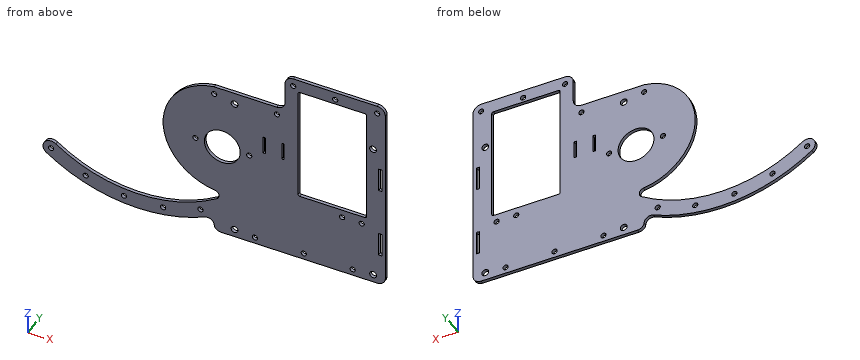
Autodesk Inventor part; units mm, degrees
ref_plane "YZ Plane" through (0, 0, 0) normal (1, 0, 0) x (0, 1, 0)
ref_plane "XZ Plane" through (0, 0, 0) normal (0, 1, 0) x (-1, 0, 0)
ref_plane "XY Plane" through (0, 0, 0) normal (0, 0, 1) x (1, 0, 0)
sketch "Sketch1" plane through (0, 0, 0) normal (0, 1, 0) x (-1, 0, 0)
  arc A0 (-0.3814, 2.9757) -> (-3, 0) centre (0, 0) ccw
  circle A1 centre (-5, 35) radius 11
  arc A2 (-0.3814, 2.9757) -> (0, 75) centre (-5, 39.0133) ccw
  line L0 (-105, 0) -> (0, 0) construction
  line L1 (-3, 0) -> (-105, 0) construction
  arc A3 (-3, 0) -> (-0.3814, -2.9757) centre (0, 0) ccw
  arc A4 (-1.6619, -2.4976) -> (97.0992, -0.9275) centre (46.5785, 70) ccw
  arc A5 (102.9008, -9.0725) -> (97.0992, -0.9275) centre (100, -5) ccw
  line L2 (0, 0) -> (100, 0) construction
  arc A6 (5.6849, -18.0476) -> (102.9008, -9.0725) centre (46.5785, 70) ccw
  line L3 (0, 75) -> (0, 0) construction
  line L4 (0, 0) -> (0, -15.1769) construction
  line L5 (0, 0) -> (-105, 0) construction
  line L6 (0, 75) -> (-105, 75)
  line L7 (-105, 75) -> (-105, -25)
  line L8 (0, -21.6754) -> (0, -21)
  line L9 (-4, -25) -> (-105, -25)
  arc A7 (5.6849, -18.0476) -> (0, -21.6754) centre (4, -21.6754) ccw
  arc A8 (-4, -25) -> (0, -21) centre (-4, -21) ccw
  point P0 (-5, -39.0133)
  point P1 (0, -25)
  dimension "d0" = 6
  dimension "d7" = 22
  dimension "d13" = 5
  dimension "d47" = 10
  dimension "d49" = 100
  dimension "d68" = 70
  dimension "d71" = 0
  dimension "d75" = 105
  dimension "d76" = 4
  dimension "d77" = 4
  dimension "d101" = 100
  dimension "d105" = 75
  dimension "d106" = 35
  dimension "d107" = 5
extrude "Extrusion1" add sketch "Sketch1" along normal blind 2
sketch "Szkic5" plane through (0, 2, 0) normal (0, 1, 0) x (1, 0, 0)
  circle A0 centre (12.5, 20) radius 2.1
  circle A1 centre (97.5, 20) radius 2.1
  circle A2 centre (12.5, -67.5) radius 2.1
  circle A3 centre (97.5, -67.5) radius 2.1
  line L0 (12.5, 20) -> (97.5, 20) construction
  line L1 (97.5, -67.5) -> (97.5, 20) construction
  line L2 (12.5, -67.5) -> (97.5, -67.5) construction
  line L3 (0, -75) -> (105, -75) construction
  line L4 (105, -75) -> (105, 25) construction
  line L5 (105, 25) -> (4, 25) construction
  line L6 (0, 21) -> (0, 21.6754) construction
  line L7 (12.5, 20) -> (12.5, -67.5) construction
  point P0 (0, 0)
  dimension "d84" = 7.5
  dimension "d85" = 7.5
  dimension "d88" = 4.2
  dimension "d89" = 85
  dimension "d109" = 87.5
extrude "Wyciągnięcie proste4" cut sketch "Szkic5" against normal up to surface (2 mm away)
sketch "Szkic6" plane through (0, 2, 0) normal (0, 1, 0) x (1, 0, 0)
  line L0 (103, -55) -> (100.9, -55)
  line L1 (100.9, -55) -> (100.9, -40)
  line L2 (100.9, -40) -> (103, -40)
  line L3 (103, -40) -> (103, -55)
  line L4 (103, -10) -> (100.9, -10)
  line L5 (100.9, -10) -> (100.9, 5)
  line L6 (100.9, 5) -> (103, 5)
  line L7 (103, 5) -> (103, -10)
  line L8 (100.9, -40) -> (100.9, -10) construction
  line L9 (100.9, -25) -> (105, -25) construction
  line L10 (105, -75) -> (105, 25) construction
  point P0 (0, 0)
  point P1 (105, 25)
  dimension "d92" = 15
  dimension "d94" = 30
  dimension "d127" = 2.1
  dimension "d128" = 2
extrude "Wyciągnięcie proste5" cut sketch "Szkic6" against normal up to surface (2 mm away)
sketch "Sketch8" plane through (0, 2, 0) normal (0, 1, 0) x (1, 0, 0)
  circle A0 centre (-11.5, -35) radius 1.6
  circle A1 centre (21.5, -35) radius 1.6
  circle A2 centre (5, -35) radius 11 construction
  line L0 (-11.5, -35) -> (21.5, -35) construction
  point P0 (0, 0)
  dimension "d110" = 33
  dimension "d111" = 3.2
extrude "Extrusion6" cut sketch "Sketch8" against normal through all
fillet "Fillet1" radius 5 1 edges at (105, 1, -25)
sketch "Sketch9" plane through (0, 2, 0) normal (0, 1, 0) x (1, 0, 0)
  line L0 (0, -75) -> (105, -75)
  line L1 (105, -75) -> (105, -98.5)
  line L2 (105, -98.5) -> (43.5, -98.5)
  line L3 (43.5, -98.5) -> (43.5, -75)
  line L4 (43.5, -75) -> (51.5, -75)
  line L5 (51.5, -75) -> (51.5, -90.5)
  line L6 (51.5, -90.5) -> (93.5, -90.5)
  line L7 (93.5, -90.5) -> (93.5, -75)
  line L8 (105, -75) -> (93.5, -75)
  point P0 (0, 0)
  dimension "d116" = 8
  dimension "d117" = 8
  dimension "d118" = 15.5
  dimension "d119" = 42
  dimension "d130" = 51.5
extrude "Extrusion7" add sketch "Sketch9" against normal up to surface (2 mm away) contours L0 L5 L6 L7 L1 L2 L3
sketch "Sketch10" plane through (0, 2, 0) normal (0, 1, 0) x (1, 0, 0)
  line L0 (93.5, -75) -> (51.5, -75)
  line L1 (51.5, -75) -> (93.5, -75)
  line L2 (93.5, -75) -> (93.5, -18)
  line L3 (93.5, -18) -> (51.5, -18)
  line L4 (51.5, -18) -> (51.5, -75)
  point P0 (0, 0)
  dimension "d123" = 57
extrude "Extrusion8" cut sketch "Sketch10" against normal up to surface (2 mm away)
fillet "Fillet2" radius 5 3 edges at (105, 1, 98.5) (43.5, 1, 98.5) (43.5, 1, 75)
fillet "Fillet3" radius 1 4 edges at (51.5, 1, 18) (93.5, 1, 18) (93.5, 1, 90.5) (51.5, 1, 90.5)
sketch "Sketch11" plane through (0, 2, 0) normal (0, 1, 0) x (1, 0, 0)
  line L0 (78.5, -13) -> (90.5, -13) construction
  line L1 (52.5, -18) -> (92.5, -18) construction
  line L2 (93.5, -19) -> (93.5, -89.5) construction
  point P0 (0, 0)
  dimension "d131" = 5
  dimension "d132" = 3
  dimension "d133" = 12
hole "Hole1" at (78.5, 2, 13) at (90.5, 2, 13) direction (0, -1, 0) diameter 3.2 end through all
sketch "Sketch12" plane through (0, 2, 0) normal (0, 1, 0) x (1, 0, 0)
  arc A0 (1.6619, 2.4976) -> (-97.0992, 0.9275) centre (-46.5785, -70) ccw construction
  arc A1 (-102.9008, 9.0725) -> (-97.0992, 0.9275) centre (-100, 5) ccw construction
  arc A2 (13.245, 0) -> (-100, 5) centre (-46.5785, -70) ccw construction
  line L0 (-46.5785, -70) -> (-100, 5) construction
  arc A3 (100, -98.5) -> (105, -93.5) centre (100, -93.5) ccw construction
  arc A4 (43.5, -93.5) -> (48.5, -98.5) centre (48.5, -93.5) ccw construction
  line L1 (25, 21) -> (85, 21) construction
  line L2 (100, 25) -> (4, 25) construction
  line L3 (48.5, -93.5) -> (100, -93.5) construction
  line L4 (0, -70) -> (38.5, -70) construction
  line L5 (0, -75) -> (38.5, -75) construction
  line L6 (38.5, -70) -> (38.5, -75) construction
  arc A5 (43.5, -80) -> (38.5, -75) centre (38.5, -80) ccw construction
  arc A6 (0.3814, -2.9757) -> (0, -75) centre (5, -39.0133) ccw construction
  line L7 (0, -75) -> (0, -70) construction
  circle A7 centre (12.5, 20) radius 2.1 construction
  circle A8 centre (97.5, 20) radius 2.1 construction
  line L8 (0, 0) -> (13.245, 0) construction
  point P0 (-78.7683, 16.2709)
  point P1 (-55.3429, 21.6626)
  point P2 (-31.3202, 20.8077)
  point P3 (-8.3374, 13.7643)
  point P4 (55, 21)
  point P5 (74.25, -93.5)
  dimension "d143" = 60
  dimension "d145" = 60
  dimension "d146" = 4
  dimension "d147" = 5
  dimension "d148" = 12.5
  dimension "d149" = 12.5
hole "Hole2" at (-100, 2, -5) at (-78.7683, 2, -16.2709) at (-55.3429, 2, -21.6626) at (-31.3202, 2, -20.8077) at (-8.3374, 2, -13.7643) at (48.5, 2, 93.5) at (100, 2, 93.5) at (25, 2, -21) at (85, 2, -21) at (55, 2, -21) at (74.25, 2, 93.5) at (0, 2, 70) at (38.5, 2, 70) direction (0, -1, 0) diameter 3.2 end through all
sketch "Sketch15" plane through (0, 2, 0) normal (0, 1, 0) x (1, 0, 0)
  line L0 (30, -40) -> (31.5, -40)
  line L1 (31.5, -40) -> (31.5, -51)
  line L2 (31.5, -51) -> (30, -51)
  line L3 (30, -51) -> (30, -40)
  line L4 (41.5, -40) -> (43, -40)
  line L5 (43, -40) -> (43, -51)
  line L6 (43, -51) -> (41.5, -51)
  line L7 (41.5, -51) -> (41.5, -40)
  point P0 (0, 0)
  dimension "d157" = 11
  dimension "d158" = 10
  dimension "d159" = 1.5
  dimension "d160" = 40
  dimension "d161" = 30
extrude "Extrusion9" cut sketch "Sketch15" against normal through all
sketch "Sketch16" plane through (0, 2, 0) normal (0, 1, 0) x (1, 0, 0)
  line L0 (43, -40) -> (43, -51)
  line L1 (43, -51) -> (41.5, -51)
  line L2 (41.5, -51) -> (41.5, -40)
  line L3 (41.5, -40) -> (43, -40)
  line L4 (31.5, -40) -> (31.5, -51)
  line L5 (31.5, -51) -> (30, -51)
  line L6 (30, -51) -> (30, -40)
  line L7 (30, -40) -> (31.5, -40)
  circle A0 centre (0, -70) radius 1.6
  circle A1 centre (55, 21) radius 1.6
  circle A2 centre (25, 21) radius 1.6
  circle A3 centre (48.5, -93.5) radius 1.6
  circle A4 centre (-31.3202, 20.8077) radius 1.6
  circle A5 centre (-78.7683, 16.2709) radius 1.6
  circle A6 centre (-100, 5) radius 1.6
  circle A7 centre (-55.3429, 21.6626) radius 1.6
  circle A8 centre (-8.3374, 13.7643) radius 1.6
  circle A9 centre (100, -93.5) radius 1.6
  circle A10 centre (85, 21) radius 1.6
  circle A11 centre (74.25, -93.5) radius 1.6
  circle A12 centre (38.5, -70) radius 1.6
  circle A13 centre (78.5, -13) radius 1.6
  circle A14 centre (90.5, -13) radius 1.6
  arc A15 (43.5, -93.5) -> (48.5, -98.5) centre (48.5, -93.5) ccw
  line L8 (48.5, -98.5) -> (100, -98.5)
  arc A16 (100, -98.5) -> (105, -93.5) centre (100, -93.5) ccw
  line L9 (105, -93.5) -> (105, 20)
  arc A17 (105, 20) -> (100, 25) centre (100, 20) ccw
  line L10 (100, 25) -> (4, 25)
  arc A18 (4, 25) -> (0, 21) centre (4, 21) ccw
  line L11 (0, 21) -> (0, 21.6754)
  arc A19 (-5.6849, 18.0476) -> (0, 21.6754) centre (-4, 21.6754) ccw
  arc A20 (-5.6849, 18.0476) -> (-102.9008, 9.0725) centre (-46.5785, -70) ccw
  arc A21 (-102.9008, 9.0725) -> (-97.0992, 0.9275) centre (-100, 5) ccw
  arc A22 (1.6619, 2.4976) -> (-97.0992, 0.9275) centre (-46.5785, -70) ccw
  arc A23 (0.3814, -2.9757) -> (1.6619, 2.4976) centre (0, 0) ccw
  arc A24 (0.3814, -2.9757) -> (0, -75) centre (5, -39.0133) ccw
  line L12 (0, -75) -> (38.5, -75)
  arc A25 (43.5, -80) -> (38.5, -75) centre (38.5, -80) ccw
  line L13 (43.5, -80) -> (43.5, -93.5)
  line L14 (93.5, -19) -> (93.5, -89.5)
  arc A26 (92.5, -90.5) -> (93.5, -89.5) centre (92.5, -89.5) ccw
  line L15 (92.5, -90.5) -> (52.5, -90.5)
  arc A27 (51.5, -89.5) -> (52.5, -90.5) centre (52.5, -89.5) ccw
  line L16 (51.5, -89.5) -> (51.5, -19)
  arc A28 (52.5, -18) -> (51.5, -19) centre (52.5, -19) ccw
  line L17 (52.5, -18) -> (92.5, -18)
  arc A29 (93.5, -19) -> (92.5, -18) centre (92.5, -19) ccw
  circle A30 centre (-11.5, -35) radius 1.6
  circle A31 centre (21.5, -35) radius 1.6
  line L18 (103, -55) -> (100.9, -55)
  line L19 (100.9, -55) -> (100.9, -40)
  line L20 (100.9, -40) -> (103, -40)
  line L21 (103, -40) -> (103, -55)
  line L22 (100.9, -10) -> (100.9, 5)
  line L23 (100.9, 5) -> (103, 5)
  line L24 (103, 5) -> (103, -10)
  line L25 (103, -10) -> (100.9, -10)
  circle A32 centre (12.5, -67.5) radius 2.1
  circle A33 centre (97.5, -67.5) radius 2.1
  circle A34 centre (97.5, 20) radius 2.1
  circle A35 centre (12.5, 20) radius 2.1
  circle A36 centre (5, -35) radius 11
sketch "Sketch17" plane through (0, 2, 0) normal (0, 1, 0) x (1, 0, 0)
  circle A0 centre (14, 7) radius 7.5
  line L0 (100, 25) -> (4, 25) construction
  line L1 (105, -93.5) -> (105, 20) construction
  circle A1 centre (32, 7) radius 7.5
  circle A2 centre (50, 7) radius 7.5
  circle A3 centre (68, 7) radius 7.5
  circle A4 centre (86, 7) radius 7.5
  line L2 (5, -35) -> (5, -13) construction
  circle A5 centre (5, -13) radius 7.5
  circle A6 centre (-14.0526, -24) radius 7.5
  circle A7 centre (-14.0526, -46) radius 7.5
  circle A8 centre (5, -57) radius 7.5
  circle A9 centre (23, -9) radius 7.5
  circle A10 centre (41, -9) radius 7.5
  point P0 (0, 0)
  dimension "d164" = 15
  dimension "d165" = 14
  dimension "d166" = 7
  dimension "d169" = 18
  dimension "d174" = 22
  dimension "d177" = 180
  dimension "d179" = 16
  dimension "d180" = 9
  dimension "d183" = 18
properties part number "wstepna_geometria_wersja_2" material "Aluminum 6061"
Design review of the part built by this model. Coordinates are the model's own, in mm. Give positions to 0.01 mm unless a question says otherwise; leave off trailing zeros. Loops run counter-clockwise (first coordinate to the right, second up) from the corner with the lowest first, then second, coordinate; pieces in that order, holes last. Notation, with made-up numbers: M 53.5,61.25 L 107.5,61.25 A18 cw 107.5,78.25 Z; hole C 23.5,-17 d6. An arc over 180 degrees is marked long. Return JSON: item names as keys, results as strings. Group by question number.
Item 1: We need section D-D (x = -36). Give the boundary of the cut face in (y, z), and give its area (3 significant figures).
Item 2: Insertion check: pin 1 Ø1.2 at (x, y) = (42.5, 1) entering from +Z; pin 2 Ø0.6 at (x, y) = (59.5, 1) entering from -Z. Each pin has a flat end and moves straight along its axis. Give the tip position at first contact, or say it passes through.
Item 3: For probe 1 along Z at (x, y) = (55, 0.65); probe 2 along X at (y, z) = (1.6, 93.5); probe 3 along Z at (x, y) = (97.5, 1.45), list the stretches that pass through material, from the lowest coordinate up.
Item 4: We need section B-B (z = 29). Give the boundary of the cut face in (x, y).
Item 5: We need section A-A (z = 87). Give the boundary of the cut face in (x, y).
Item 6: We need section C-C (z = 57). Give the boundary of the cut face in (x, y).
Output:
{
 "1": {"outline": "M 0,-26.5 L 2,-26.5 L 2,-16.44 L 0,-16.44 Z", "area": "20.1 mm^2"},
 "2": {"pin 1": "stops at z = 78.04", "pin 2": "stops at z = -25"},
 "3": {"probe 1": "z = -25 to -22.6, -19.4 to 18, 90.5 to 98.5", "probe 2": "x = 43.5 to 46.9, 50.1 to 72.65, 75.85 to 98.4, 101.6 to 105", "probe 3": "z = -25 to -22.1, -17.9 to 65.4, 69.6 to 98.5"},
 "4": {"outline": "M -29.93,0 L -4.22,0 L -4.22,2 L -29.93,2 Z; M 14.22,0 L 51.5,0 L 51.5,2 L 14.22,2 Z; M 93.5,0 L 105,0 L 105,2 L 93.5,2 Z"},
 "5": {"outline": "M 43.5,0 L 51.5,0 L 51.5,2 L 43.5,2 Z; M 93.5,0 L 105,0 L 105,2 L 93.5,2 Z"},
 "6": {"outline": "M -26.57,0 L 51.5,0 L 51.5,2 L -26.57,2 Z; M 93.5,0 L 105,0 L 105,2 L 93.5,2 Z"}
}
